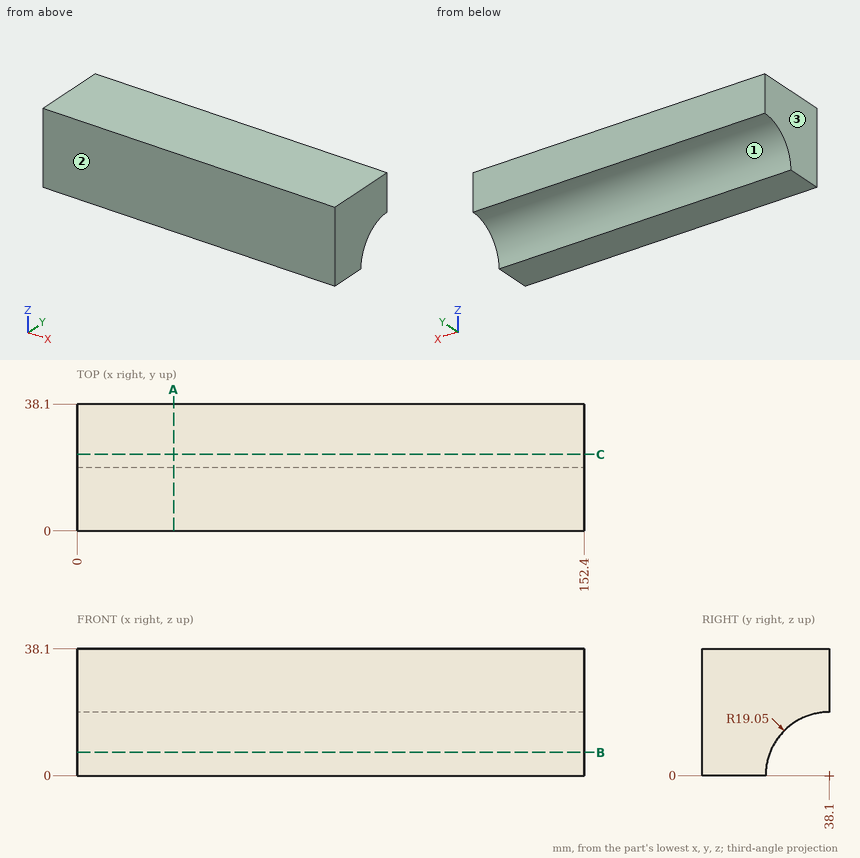
Source: three-view drawing plus pictorial views. Frame: mm from the lowest corner of the part. Give positions to 0.01 mm unless a question says otherwise; leave off trailing zeros. Loops run counter-clockwise (first coordinate to the right, second up) from the corner with the lowest first, then second, coordinate; pieces in that order, holes last. Notation, with made-up numbers: (55.25, 19) -> (62.25, 19) arc R15 ccw to (62.25, 44) -> close; hole circle Ø5 at (76, 16.5). An arc over 180 degrees is marked (long way). Use a Markdown table: item, result. Add a question column.
(1) Section query B-B (z = 7). Output: boundary loops of the cut face in (x, y), then the cut area to 3 significant figures.
(2) Ray query, line 1 (Y direction, x = 45, z = 6); line 2 (Z direction, x = 62.5, y = 25.5); line 3 (Z direction, x = 81.5, y = 22). Return the intervals inside material, ascending.
(3) Section query C-C (y = 23). Output: boundary loops of the cut face in (x, z), then the cut area to 3 significant figures.
(4) Pull-direction query (Y, two-part tool) for the marked faces 1, 2 and 3; classes: +Y half, -Y half, draft (parallel to the pull), parting line (faces both ways), or undercut.
(5) First-contact query: pin 1 Ø5 at (x, z) = (57, 5) entering from +Y. Flat tip, straight axial feed; report the tip coordinate or a pass-through.
(6) Section query A-A (x = 29). Output: boundary loops of the cut face in (y, z).
Checked values:
| question | item | result |
|---|---|---|
| 1 | outline | (0, 0) -> (152.4, 0) -> (152.4, 20.38) -> (0, 20.38) -> close |
| 1 | area | 3,110 mm^2 |
| 2 | line 1 | 0 to 20.02 |
| 2 | line 2 | 14.29 to 38.1 |
| 2 | line 3 | 10.18 to 38.1 |
| 3 | outline | (0, 11.61) -> (152.4, 11.61) -> (152.4, 38.1) -> (0, 38.1) -> close |
| 3 | area | 4,040 mm^2 |
| 4 | face 1 | +Y half |
| 4 | face 2 | -Y half |
| 4 | face 3 | draft |
| 5 | pin 1 | y = 20.59 |
| 6 | outline | (0, 0) -> (19.05, 0) arc R19.05 cw to (38.1, 19.05) -> (38.1, 38.1) -> (0, 38.1) -> close |
